Autodesk Inventor part; units mm, degrees
ref_plane "YZ Plane" through (0, 0, 0) normal (1, 0, 0) x (0, 1, 0)
ref_plane "XZ Plane" through (0, 0, 0) normal (0, 1, 0) x (-1, 0, 0)
ref_plane "XY Plane" through (0, 0, 0) normal (0, 0, 1) x (1, 0, 0)
sketch "Sketch1" plane through (0, 0, 0) normal (0, 0, 1) x (1, 0, 0)
  circle A0 centre (10, 11.5) radius 0.5
  line L0 (0, 0) -> (20.0001, 0)
  line L1 (0, 0) -> (0, 3)
  line L2 (20.0001, 0) -> (20.0001, 3)
  line L3 (0, 3) -> (16, 3) construction
  line L4 (20.0001, 3) -> (36.0001, 3) construction
  arc A1 (14.3301, 14) -> (5.6699, 14) centre (10, 11.5) ccw
  line L5 (10, 11.5) -> (5.6699, 14) construction
  line L6 (10, 11.5) -> (14.3301, 14) construction
  line L7 (5.6699, 14) -> (0, 3)
  line L8 (14.3301, 14) -> (20.0001, 3)
  dimension "d17" = 3
  dimension "d18" = 3
  dimension "d19" = 11.5
  dimension "d23" = 90
  dimension "d24" = 90
  dimension "d25" = 10
  dimension "d31" = 5
  dimension "d32" = 120
  dimension "d33" = 14
  dimension "d48" = 1
extrude "Extrusion1" add sketch "Sketch1" along normal blind 4.5
sketch "Sketch4" plane through (0, 0, 4.5) normal (0, 0, 1) x (1, 0, 0)
  line L0 (0, 3) -> (0, 0)
  line L1 (20.0001, 0) -> (20.0001, 3)
  line L2 (0, 0) -> (20.0001, 0)
  line L3 (20.0001, 0) -> (20.0001, 3)
  line L4 (20.0001, 3) -> (0, 3)
  line L5 (0, 3) -> (0, 0)
extrude "Extrusion2" add sketch "Sketch4" along normal blind 4.5
sketch "Sketch5" plane through (0, 0, 0) normal (0, -1, 0) x (1, 0, 0)
  circle A0 centre (5, 4.8) radius 1.6
  circle A1 centre (15, 4.8) radius 1.6
  line L0 (0, 0) -> (20.0001, 0)
  dimension "d13" = 3.2
  dimension "d14" = 3.2
  dimension "d38" = 4.8
  dimension "d39" = 4.8
extrude "Extrusion3" cut sketch "Sketch5" against normal through all
sketch "Sketch6" plane through (0, 3, 9) normal (0, 1, 0) x (1, 0, 0)
  circle A0 centre (5, 4.2) radius 1.6
  circle A1 centre (5, 4.2) radius 3
  circle A2 centre (15, 4.2) radius 1.6
  circle A3 centre (15, 4.2) radius 3
  line L0 (0, 9) -> (20.0001, 9)
  dimension "d34" = 6
  dimension "d35" = 6
  dimension "d40" = 4.8
  dimension "d41" = 4.8
extrude "Extrusion4" cut sketch "Sketch6" along normal up to next
sketch "Sketch7" plane through (0, 0, 0) normal (0, -1, 0) x (1, 0, 0)
  line L0 (0, 0) -> (0, 9)
  line L1 (2.042, 0) -> (0, 0)
  line L2 (0, 0) -> (0, 9)
  line L3 (0, 9) -> (2.042, 9)
  line L4 (2.042, 9) -> (2.042, 0)
extrude "Extrusion5" cut sketch "Sketch7" against normal up to next
sketch "Sketch8" plane through (20.0001, 0, 0) normal (0, -1, 0) x (1, 0, 0)
  line L0 (0, 4.5) -> (0, 9)
  line L1 (-2.042, 0) -> (0, 0)
  line L2 (0, 0) -> (0, 9)
  line L3 (0, 9) -> (-2.042, 9)
  line L4 (-2.042, 9) -> (-2.042, 0)
  point P0 (-20.0001, 0)
extrude "Extrusion6" cut sketch "Sketch8" against normal up to next
properties part number "lower_deck_shaft_mount_printing"
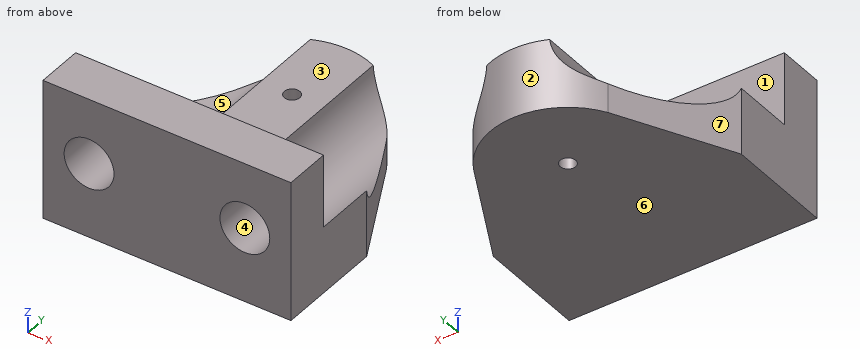
The model under review builds one solid part; all positions refer to its coordinate system, in mm. Face numbers are marked on the shaded views. A direction names the side the tool comes from. Coordinates: 2 decimals unless noted, no trailing zeros. Write each loop counter-clockwise with the first axis right and the second up, starting at its lowest first coordinate (ties: lowest second). Pieces come first, ordered by that corner, then holes.
1) Clearance check with flat-ended pins moving along their axes: pin 1 Ø1 at (x, y) = (7, 10) entering from +Z; pin 2 Ø3 at (y, z) = (13.5, 1.5) entering from -X; pin 3 Ø1 at (y, z) = (8, 2.5) entering from +X. State where each tip first meets the part, or that it passes through.
2) To check wall thickness, follow probe 1 along Y at (x, z) = (4.5, 6.75); probe 2 along Z at (x, y) = (5, 0.9); probe 3 along Z at (x, y) = (9.75, 9). State the ranges of each line that lie inside material, in increasing order.
3) The part is to be moulded in two halves that separate along Z. For the marked faces 4, 5, 6 and 7, say which applies: pulls with the +Z half, pulls with the -Z half, needs draft (parallel to the pull), parting line crosses it, or undercut.
4) We need section B-B on z = 4.8. State the section outline as (x, y) points.
5) Machinability: for the marked faces 1, 2 and 3, which of the approach directions +Z, -Z, +X, -X, +Y, -Y give a long, thin tool a straight path to every point of the face, cutting with its end or side? Answer none if there is none.
6) We need section A-A on x = 10. State the section outline as (y, z) points.
7) We need section C-C on y = 11.5. State the section outline as (x, z) points, then the cut area to 3 significant figures.
8) We need section D-D on y = 6.25. State the section outline as (x, z) points, then the cut area to 3 significant figures.
Answer list:
1. pin 1: stops at z = 3.14
1. pin 2: stops at x = 4.64
1. pin 3: stops at x = 17.68
2. probe 1: y = 0 to 3
2. probe 2: z = 0 to 3.2, 6.4 to 9
2. probe 3: z = 0 to 4.5
3. face 4: undercut
3. face 5: pulls with the +Z half
3. face 6: pulls with the -Z half
3. face 7: needs draft
4. outline: (2.04, 0) - (3.4, 0) - (3.4, 3) - (2.04, 3) - close; (6.6, 0) - (13.4, 0) - (13.4, 3) - (6.6, 3) - close; (16.6, 0) - (17.96, 0) - (17.96, 3) - (16.6, 3) - close
5. face 1: +Z, +Y
5. face 2: +Z, -Z, +Y
5. face 3: +Z, +X, -X, +Y
6. outline: (0, 0) - (11, 0) - (11, 4.5) - (3, 4.5) - (3, 9) - (0, 9) - close; (12, 0) - (16.5, 0) - (16.5, 4.5) - (12, 4.5) - close
7. outline: (4.38, 0) - (9.5, 0) - (9.5, 4.5) - (7.98, 4.5) arc R3 cw to (4.38, 1.86) - close; (10.5, 0) - (15.62, 0) - (15.62, 1.86) arc R3 cw to (12.02, 4.5) - (10.5, 4.5) - close
7. area: 30.4 mm2
8. outline: (2.04, 0) - (17.96, 0) - (17.96, 4.3) arc R3 cw to (12.02, 4.5) - (7.98, 4.5) arc R3 cw to (2.04, 4.3) - close
8. area: 46.9 mm2
